Geometry check sheet. Reference: the model listing, model coordinates, mm. Face numbers are marked on the shaded views. A direction names the side the tool comes from. Round coordinates to 2 decimals unless told otherwise and drop trailing zeros. Order: outer loops, then holes, each group sorted by start corner. A loop starts at its lowest first (then second) coordinate and runs counter-clockwise, first axis right, second up.
```python
from build123d import *

# Parameters (mm, degrees)
F1_DEPTH  = 46.99
F2_T      = -3.175
F5_DEPTH  = 12.7
F6_R      = 635
F7_DEPTH  = 279.4
F8_DEPTH  = 3.175
F9_W      = 137.16
F9_H      = 3.175
F10_DEPTH = 19.05


# Not quite as in the source:
# - a feature names something its author has since deleted; it is built from what else it names


with BuildPart() as f1:
    # F0 (on Front) → F1 (new body)
    with BuildSketch(Plane.XZ):
        Polygon((-72.39, 53.975), (-81.28, 53.975), (-81.28, 45.085), (-81.28, -45.085), (-81.28, -53.975), (-72.39, -53.975), (72.39, -53.975), (81.28, -53.975), (81.28, -45.085), (81.28, 45.085), (81.28, 53.975), (72.39, 53.975), align=None)
    extrude(amount=F1_DEPTH)

    # F2
    f2_openings = [f1.faces().sort_by_distance(p)[0] for p in [
        (0, 0, 0),
    ]]
    offset(amount=F2_T, openings=f2_openings)

    # F0 (on Front) → F5 (join)
    with BuildSketch(Plane.XZ):
        with BuildLine():
            Line((-81.28, 45.085), (-81.28, 53.975))
            Line((-81.28, 53.975), (-72.39, 53.975))
            ThreePointArc((-72.39, 53.975), (-87.5661792847, 60.2611792847), (-81.28, 45.085))
        make_face()
        with BuildLine():
            Line((-81.28, -53.975), (-81.28, -45.085))
            ThreePointArc((-81.28, -45.085), (-87.5661792847, -60.2611792847), (-72.39, -53.975))
            Line((-72.39, -53.975), (-81.28, -53.975))
        make_face()
        with BuildLine():
            ThreePointArc((81.28, 45.085), (87.5661792847, 60.2611792847), (72.39, 53.975))
            Line((72.39, 53.975), (81.28, 53.975))
            Line((81.28, 53.975), (81.28, 45.085))
        make_face()
        with BuildLine():
            ThreePointArc((72.39, -53.975), (87.5661792847, -60.2611792847), (81.28, -45.085))
            Line((81.28, -45.085), (81.28, -53.975))
            Line((81.28, -53.975), (72.39, -53.975))
        make_face()
    extrude(amount=F5_DEPTH)

    # F6 (on offset) → F7 (cut)
    with BuildSketch(Plane(origin=(-106.68, 0, 0), x_dir=(0, -1, 0), z_dir=(-1, 0, 0))):
        with Locations((-630.555, 0)):
            Circle(F6_R)
    extrude(amount=-F7_DEPTH, mode=Mode.SUBTRACT)

    # F4 (on face) → F8 (cut)
    with BuildSketch(Plane(origin=(-81.28, 0, 0), x_dir=(0, -1, 0), z_dir=(-1, 0, 0))):
        Polygon((24.13, 0), (13.97, 0), (3.81, 0), (3.81, -6.35), (24.13, -6.35), align=None)
        Polygon((3.81, 0), (13.97, 0), (24.13, 0), (24.13, 6.35), (3.81, 6.35), align=None)
    extrude(amount=-F8_DEPTH, mode=Mode.SUBTRACT)

    # F9 (on face) → F10 (join)
    with BuildSketch(Plane(origin=(0, -43.815, 0), x_dir=(-1, 0, 0), z_dir=(0, 1, 0))):
        with Locations((-9.525, -1.5875)):
            Rectangle(F9_W, F9_H)
        with Locations((-9.525, 1.5875)):
            Rectangle(F9_W, F9_H)
    extrude(amount=F10_DEPTH)


solid = f1.part
```
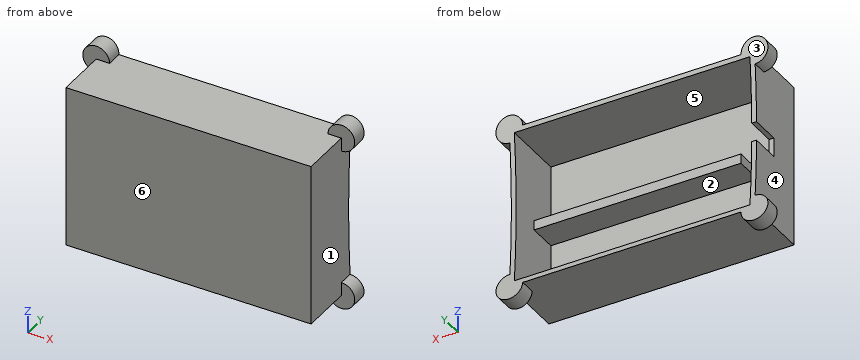
(1) Depth check by flat-ended pin: P1, Ø3, axis at x = -14.5, y = -29, coming from the +Z side (3 decimals); P2, Ø2, axis at y = -29, z = 28.5, coming from the -X side; P3, Ø4, axis at x = -16.5, z = 15.5, coming from the +Y side (3 decimals). Enter the tip coordinate at first touch or a pass-through.
Returned:
P1: stops at z = 53.975
P2: stops at x = -81.28
P3: stops at y = -43.815
(2) Set-up check for the marked faces 1, 2 and 3: record each of +Z, -Z, +X, -X, +Y, -Y from which the full face is reachable in a straight line by a thin tool's end or side.
Returned:
face 1: +X, -Y
face 2: +Y
face 3: +X, -X, +Y
(3) Draft check along X on the marked faces 4, 5 and 6. Enter one of: released by +X, released by -X, zero draft, split by the parting line, or undercut.
Returned:
face 4: released by -X
face 5: undercut
face 6: zero draft
(4) Sectioned sample at A-A, the plane y = -34. Record the cut outline in (x, z) (3 decimals), and give its area (3 significant figures).
Returned:
outline: (-81.28, -53.975) - (81.28, -53.975) - (81.28, 53.975) - (-81.28, 53.975) - close; hole (-78.105, -50.8) - (78.105, -50.8) - (78.105, -3.175) - (-59.055, -3.175) - (-59.055, 3.175) - (78.105, 3.175) - (78.105, 50.8) - (-78.105, 50.8) - close
area: 2,550 mm2
(5) Sectioned sample at C-C, the plane x = -63. Record the cut outline in (y, z) (3 decimals), and give its area (3 significant figures).
Returned:
outline: (-46.99, -53.975) - (-2.147, -53.975) arc R635 cw to (-2.41, -50.8) - (-43.815, -50.8) - (-43.815, 50.8) - (-2.41, 50.8) arc R635 cw to (-2.147, 53.975) - (-46.99, 53.975) - close
area: 606 mm2
(6) Sectioned sample at D-D, the plane z = -23.5. Record the cut outline in (x, y) (3 decimals), and give its area (3 significant figures).
Returned:
outline: (-81.28, -46.99) - (81.28, -46.99) - (81.28, -4.01) - (78.105, -4.01) - (78.105, -43.815) - (-78.105, -43.815) - (-78.105, -4.01) - (-81.28, -4.01) - close
area: 769 mm2
(7) Sectioned sample at B-B, the plane y = -16.5. Record the cut outline in (x, z) (3 decimals).
Returned:
outline: (-81.28, -53.975) - (81.28, -53.975) - (81.28, 53.975) - (-81.28, 53.975) - (-81.28, 6.35) - (-78.105, 6.35) - (-78.105, 50.8) - (78.105, 50.8) - (78.105, -50.8) - (-78.105, -50.8) - (-78.105, -6.35) - (-81.28, -6.35) - close
(8) Material ranges on line 1 (Z direction, x = 33, y = -26) (3 decimals); line 2 (Z direction, x = -77, y = -14) (3 decimals); line 3 (X direction, y = -7, z = -38) (3 decimals), recorded low to high.
Returned:
line 1: z = -53.975 to -50.8, -3.175 to 3.175, 50.8 to 53.975
line 2: z = -53.975 to -50.8, 50.8 to 53.975
line 3: x = -81.28 to -78.105, 78.105 to 81.28
